from build123d import *

# Parameters (mm, degrees)
SKETCH1_R           = 2.4892
SKETCH1_R_2         = 14.2875
BOSS_EXTRUDE1_DEPTH = 3.175
FILLET1_R           = 6.35


with BuildPart() as part:
    # Sketch1 → Boss-Extrude1 (new, symmetric)
    with BuildSketch(Plane(origin=(0, 0, 0), x_dir=(0, 0, -1), z_dir=(1, 0, 0))):
        with BuildLine():
            Line((21.078264706, -21.575058824), (30.1625, -12.7))
            Line((30.1625, -12.7), (87.3125, -12.7))
            Line((87.3125, -12.7), (87.3125, 12.7))
            Line((87.3125, 12.7), (30.1625, 12.7))
            Line((30.1625, 12.7), (21.078264706, 21.575058824))
            ThreePointArc((21.078264706, 21.575058824), (-30.1625, 0), (21.078264706, -21.575058824))
        make_face()
        with Locations((55.5625, 0)):
            Circle(SKETCH1_R, mode=Mode.SUBTRACT)
        with Locations((68.2625, 0)):
            Circle(SKETCH1_R, mode=Mode.SUBTRACT)
        with Locations((-11.90625, 20.622229928)):
            Circle(SKETCH1_R, mode=Mode.SUBTRACT)
        with Locations((11.90625, 20.622229928)):
            Circle(SKETCH1_R, mode=Mode.SUBTRACT)
        with Locations((-11.90625, -20.622229928)):
            Circle(SKETCH1_R, mode=Mode.SUBTRACT)
        with Locations((11.90625, -20.622229928)):
            Circle(SKETCH1_R, mode=Mode.SUBTRACT)
        with Locations((-23.8125, 0)):
            Circle(SKETCH1_R, mode=Mode.SUBTRACT)
        Circle(SKETCH1_R_2, mode=Mode.SUBTRACT)
        with Locations((23.8125, 0)):
            Circle(SKETCH1_R, mode=Mode.SUBTRACT)
    extrude(amount=BOSS_EXTRUDE1_DEPTH, both=True)

    # Fillet1
    fillet1_edges = [part.edges().sort_by_distance(p)[0] for p in [
        (0, 12.7, -30.1625),
        (0, 12.7, -87.3125),
        (0, -12.7, -87.3125),
        (0, -12.7, -30.1625),
    ]]
    fillet(fillet1_edges, radius=FILLET1_R)


solid = part.part
The model under review builds one solid part; all positions refer to its coordinate system, in mm. Give positions to 0.01 mm unless a question says otherwise; leave off trailing zeros. Write each loop counter-clockwise with the first axis right and the second up, starting at its lowest first coordinate (ties: lowest second). Pieces come first, ordered by that corner, then holes. Notation, with made-up numbers: M 56,87.25 L 73,87.25 A24 cw 73,100.25 Z; hole C 12,14.5 d9. An arc over 180 degrees is marked long. One line per question, with ' | ' between items. Start each with the question number.
Item 1: We need section D-D on z = -40. Write out the cut boundary in (x, y) (3 decimals), plus the area to 3 significant figures.
Item 2: Wall thickness on line 1 (Y direction, x = -1.5, z = 0); line 2 (Z direction, x = -1.5, y = 22); line 3 (Y direction, x = 0.75, z = -37): over which ranges is each line inside the solid? List them lowest first. Write a range as from..to.
Item 3: We need section A-A on y = 5. Write out the cut boundary in (x, z) (1 decimal), plus the area to 3 significant figures.
Item 4: We need section B-B on z = 0. Write out the cut boundary in (x, y) (1 decimal), plus the area to 3 significant figures.
Item 5: We need section C-C on x = 0.5. Give the number of separate pieces and of enclosed holes in the cut face, plus the area to 3 significant figures.
Item 6: Draft analysis for pull direction Y (two halves, no side actions). For faces 1 (the cylindrical face through (0.04, 10.89, -85.4)), 2 (the flat face through (0, 0, -87.312)), 3 (the flat face through (0.044, -18.091, -24.644)), 4 (the cylindrical face through (-0.04, -22.83, 10.76)), state which applies: released by +Y, released by -Y, zero draft, split by the parting line, or undercut.
Item 7: For pin 1 (6.5 mm diameter, centred on y = 20.62, z = -11.91, fed in from +X) (3 decimals); pin 2 (1.9 mm diameter, centred on x = -1, z = -65, fed in from +Y); pin 3 (1 mm diameter, centred on x = 1.5, z = -54, fed in from -Y); pin 4 (1 mm diameter, centred on x = -1.5, y = 15.5, fed in from -Z), all flat-tipped, find the tip position at first contact; note any pin that passes through.
Results found:
1) outline: M -3.175,-12.7 L 3.175,-12.7 L 3.175,12.7 L -3.175,12.7 Z | area: 161 mm2
2) line 1: y = -30.16..-14.29, 14.29..30.16 | line 2: z = -20.63..-13.98, -9.83..9.83, 13.98..20.63 | line 3: y = -12.7..12.7
3) outline: M -3.2,-87.3 L 3.2,-87.3 L 3.2,-13.4 L -3.2,-13.4 Z; M -3.2,13.4 L 3.2,13.4 L 3.2,29.7 L -3.2,29.7 Z | area: 573 mm2
4) outline: M -3.2,-30.2 L 3.2,-30.2 L 3.2,-14.3 L -3.2,-14.3 Z; M -3.2,14.3 L 3.2,14.3 L 3.2,30.2 L -3.2,30.2 Z | area: 202 mm2
5) separate pieces: 1 | enclosed holes: 9 | area: 3,540 mm2
6) face 1: released by +Y | face 2: zero draft | face 3: released by -Y | face 4: undercut
7) pin 1: stops at x = 3.175 | pin 2: stops at y = 12.7 | pin 3: stops at y = -12.7 | pin 4: stops at z = -27.81
